```python
from build123d import *

# Parameters (mm, degrees)
SKETCH1_W           = 101
SKETCH1_H           = 59.932047928
SKETCH1_R           = 11
SKETCH1_R_2         = 10
BOSS_EXTRUDE1_DEPTH = 10
SKETCH2_R           = 17
CUT_EXTRUDE1_DEPTH  = 10


with BuildPart() as part:
    # Sketch1 → Boss-Extrude1 (new body)
    with BuildSketch(Plane(origin=(0, 0, 0), x_dir=(1, 0, 0), z_dir=(0, 1, 0))):
        Rectangle(SKETCH1_W, SKETCH1_H)
        with Locations(Location((-20.5, 0, 0), (0, 0, 270))):
            Circle(SKETCH1_R, mode=Mode.SUBTRACT)
        with Locations(Location((20.5, 0, 0), (0, 0, 270))):
            Circle(SKETCH1_R_2, mode=Mode.SUBTRACT)
    extrude(amount=BOSS_EXTRUDE1_DEPTH)

    # Sketch2 → Cut-Extrude1 (cut)
    with BuildSketch(Plane(origin=(0, 10, 0), x_dir=(1, 0, 0), z_dir=(0, 1, 0))):
        with Locations(Location((-20.5, 0, 0), (0, 0, 270))):
            Circle(SKETCH2_R)
    extrude(amount=-CUT_EXTRUDE1_DEPTH, mode=Mode.SUBTRACT)


solid = part.part
```
Check sheet for the modelled part. Datum: model origin and axes. Units: mm. Round coordinates to 2 decimals unless told otherwise and drop trailing zeros. Order: outer loops, then holes, each group sorted by start corner. A loop starts at its lowest first (then second) coordinate and runs counter-clockwise, first axis right, second up. Notation, with made-up numbers: M 86.5,30 L 108.5,30 A32 cw 108.5,69 Z; hole C 37.5,-23.5 d5. An arc over 180 degrees is marked long. Answer in a Markdown table with one row per item.
(1) Section check C-C on y = 3.5. Record the boundary of the cut face in (x, z).
Findings:
| item | result |
|---|---|
| outline | M -50.5,-29.97 L 50.5,-29.97 L 50.5,29.97 L -50.5,29.97 Z; hole C -20.5,0 d34; hole C 20.5,0 d20 |
(2) Section check B-B on z = 0. Record the boundary of the cut face in (x, y).
Findings:
| item | result |
|---|---|
| outline | M -50.5,0 L -37.5,0 L -37.5,10 L -50.5,10 Z; M -3.5,0 L 10.5,0 L 10.5,10 L -3.5,10 Z; M 30.5,0 L 50.5,0 L 50.5,10 L 30.5,10 Z |
(3) Section check A-A on x = -20.5. Record the boundary of the cut face in (y, z), plus the area to 3 significant figures.
Findings:
| item | result |
|---|---|
| outline | M 0,-29.97 L 10,-29.97 L 10,-17 L 0,-17 Z; M 0,17 L 10,17 L 10,29.97 L 0,29.97 Z |
| area | 259 mm^2 |
(4) Section check D-D on x = 20.5. Record the boundary of the cut face in (y, z).
Findings:
| item | result |
|---|---|
| outline | M 0,-29.97 L 10,-29.97 L 10,-10 L 0,-10 Z; M 0,10 L 10,10 L 10,29.97 L 0,29.97 Z |
(5) Material ranges on line 1 along X through (y, z) = (4.25, 0); line 2 along X through (y, z) = (2.25, 4.5); line 3 along Z through (x, y) = (-35.5, 3), recorded low to high. Write a range as from..to.
Findings:
| item | result |
|---|---|
| line 1 | x = -50.5..-37.5, -3.5..10.5, 30.5..50.5 |
| line 2 | x = -50.5..-36.89, -4.11..11.57, 29.43..50.5 |
| line 3 | z = -29.97..-8, 8..29.97 |
